Geometry: final body of the model. Coordinates: model frame, mm. Face numbers are marked on the shaded views. A direction names the side the tool comes from. Give positions to 0.01 mm unless a question says otherwise; leave off trailing zeros. Write each loop counter-clockwise with the first axis right and the second up, starting at its lowest first coordinate (ties: lowest second). Pieces come first, ordered by that corner, then holes. Notation, with made-up numbers: M 17.25,82 L 62.25,82 A26 ccw 62.25,117 Z; hole C 33,35 d9. An arc over 180 degrees is marked long. Use a Markdown table: item, result. Add a question column.
(1) Material intervals for L1, parallel to Z at x = 4, y = 8.5; L2, parallel to Z at x = 1.75, y = -1.75; L3, parallel to Y at x = -1, z = 48, sorted ascending.
(2) Cut plane A-A (y = 0). Output: boundary loops of the cut face in (x, z).
(3) Reachability of the marked faces 1, 2 and 3 from +Z, -Z, +X, -X, +Y, -Y: full face, straight path, thin tool, end or side. Return the list, or none.
(4) Pin query (flat end, axial travel): pin 1 Ø4 at (x, z) = (-4.5, 21) entering from -Y; pin 2 Ø4 at (x, y) = (2.5, 2.5) entering from +Z; pin 3 Ø3 at (x, y) = (3, -1.5) entering from -Z; pin 4 Ø8 at (x, z) = (-6, 43.5) entering from -Y. Return the tip coordinate at first contact, or that it passes through.
(5) Cut plane C-C (z = 10). Output: boundary loops of the cut face in (x, y), plus the area to 3 significant figures.
(6) Cut plane D-D (x = -4). Output: boundary loops of the cut face in (y, z).
(7) Cut plane B-B (x = 0). Output: boundary loops of the cut face in (y, z), plus the area to 3 significant figures.
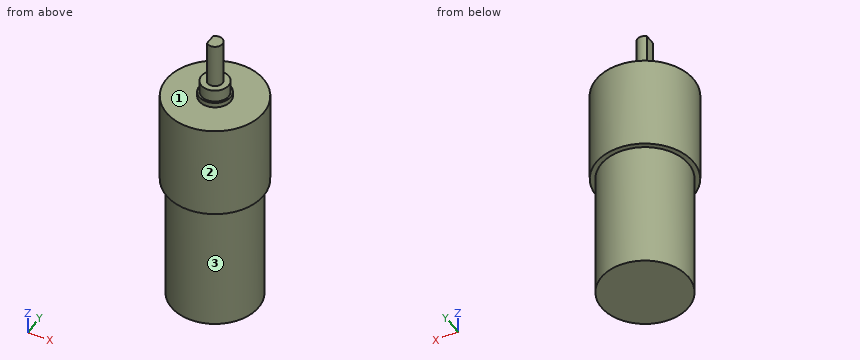
```python
from build123d import *

# Parameters (mm, degrees)
SKETCH1_R           = 8.75
BOSS_EXTRUDE1_DEPTH = 26
SKETCH2_R           = 9.75
BOSS_EXTRUDE2_DEPTH = 19
SKETCH3_R           = 3.15
BOSS_EXTRUDE3_DEPTH = 1
SKETCH4_R           = 2.75
BOSS_EXTRUDE4_DEPTH = 2.5
BOSS_EXTRUDE5_DEPTH = 9


with BuildPart() as part:
    # Sketch1 → Boss-Extrude1 (new body)
    with BuildSketch(Plane.XY):
        with Locations(Location((0, 0, 0), (0, 0, 180))):
            Circle(SKETCH1_R)
    extrude(amount=BOSS_EXTRUDE1_DEPTH)

    # Sketch2 → Boss-Extrude2 (add)
    with BuildSketch(Plane.XY.offset(26)):
        Circle(SKETCH2_R)
    extrude(amount=BOSS_EXTRUDE2_DEPTH)

    # Sketch3 → Boss-Extrude3 (add)
    with BuildSketch(Plane.XY.offset(45)):
        Circle(SKETCH3_R)
    extrude(amount=BOSS_EXTRUDE3_DEPTH)

    # Sketch4 → Boss-Extrude4 (add)
    with BuildSketch(Plane.XY.offset(46)):
        Circle(SKETCH4_R)
    extrude(amount=BOSS_EXTRUDE4_DEPTH)

    # Sketch5 → Boss-Extrude5 (add)
    with BuildSketch(Plane.XY.offset(48.5)):
        with BuildLine():
            Line((-1, 1.118033989), (-1, -1.118033989))
            ThreePointArc((-1, -1.118033989), (1.5, 0), (-1, 1.118033989))
        make_face()
    extrude(amount=BOSS_EXTRUDE5_DEPTH)


solid = part.part
```
Answer list:
| question | item | result |
|---|---|---|
| 1 | L1 | 26 to 45 |
| 1 | L2 | 0 to 48.5 |
| 1 | L3 | -2.56 to 2.56 |
| 2 | outline | M -9.75,26 L -8.75,26 L -8.75,0 L 8.75,0 L 8.75,26 L 9.75,26 L 9.75,45 L 3.15,45 L 3.15,46 L 2.75,46 L 2.75,48.5 L 1.5,48.5 L 1.5,57.5 L -1,57.5 L -1,48.5 L -2.75,48.5 L -2.75,46 L -3.15,46 L -3.15,45 L -9.75,45 Z |
| 3 | face 1 | +Z |
| 3 | face 2 | +Z, -Z |
| 3 | face 3 | -Z |
| 4 | pin 1 | y = -8.39 |
| 4 | pin 2 | z = 48.5 |
| 4 | pin 3 | z = 0 |
| 4 | pin 4 | y = -9.54 |
| 5 | outline | C 0,0 d17.5 |
| 5 | area | 241 mm² |
| 6 | outline | M -8.89,26 L -7.78,26 L -7.78,0 L 7.78,0 L 7.78,26 L 8.89,26 L 8.89,45 L -8.89,45 Z |
| 7 | outline | M -9.75,26 L -8.75,26 L -8.75,0 L 8.75,0 L 8.75,26 L 9.75,26 L 9.75,45 L 3.15,45 L 3.15,46 L 2.75,46 L 2.75,48.5 L 1.5,48.5 L 1.5,57.5 L -1.5,57.5 L -1.5,48.5 L -2.75,48.5 L -2.75,46 L -3.15,46 L -3.15,45 L -9.75,45 Z |
| 7 | area | 873 mm² |
